from build123d import *

# Parameters (mm, degrees)
F0_R      = 2.0455133379
F0_R_2    = 1.5
F1_DEPTH  = 20
F0_W      = 30
F0_H      = 6.4
F2_DEPTH  = 30
F3_R      = 6.5
F4_DEPTH  = 18.001
F5_R      = 3
F5_R_2    = 2.0455133379
F6_DEPTH  = 15
F7_R      = 9.25
F8_DEPTH  = 20.001
F9_DEPTH  = 10
F11_DEPTH = 3


with BuildPart() as f1:
    # F0 (on Top) → F1 (new body)
    with BuildSketch(Plane.XY):
        Polygon((11.3, 6.4), (0, 6.4), (-27.3, 6.4), (-27.3, -6.4), (-11, -6.4), (-11, -4.4), (0, -4.4), (11, -4.4), (11, -6.4), (27.3, -6.4), (27.3, 0), (27.3, 13.6), (11.3, 13.6), align=None)
        with Locations((-21, -0.9)):
            Circle(F0_R, mode=Mode.SUBTRACT)
        with Locations((-9, 1.4)):
            Circle(F0_R_2, mode=Mode.SUBTRACT)
        with Locations((9, 1.4)):
            Circle(F0_R_2, mode=Mode.SUBTRACT)
        with Locations((21, -0.9)):
            Circle(F0_R, mode=Mode.SUBTRACT)
    extrude(amount=F1_DEPTH)

    # F0 (on Top) → F2 (join)
    with BuildSketch(Plane.XY):
        with Locations((42.3, -3.2)):
            Rectangle(F0_W, F0_H)
    extrude(amount=F2_DEPTH)

    # F3 (on face) → F4 (cut, through all)
    with BuildSketch(Plane.XZ.offset(4.4)):
        with Locations((0, 20)):
            Circle(F3_R)
    extrude(amount=-F4_DEPTH, mode=Mode.SUBTRACT)

    # F5 (on face) → F6 (cut)
    with BuildSketch(Plane(origin=(0, 0, 0), x_dir=(1, 0, 0), z_dir=(0, 0, -1))):
        with Locations((-21, 0.9)):
            Circle(F5_R)
        with Locations((-21, 0.9)):
            Circle(F5_R_2, mode=Mode.SUBTRACT)
        with Locations((21, 0.9)):
            Circle(F5_R)
        with Locations((21, 0.9)):
            Circle(F5_R_2, mode=Mode.SUBTRACT)
    extrude(amount=-F6_DEPTH, mode=Mode.SUBTRACT)

    # F7 (on face) → F8 (cut, through all)
    with BuildSketch(Plane.XZ.offset(6.4)):
        with Locations((42.3, 15)):
            Circle(F7_R)
    extrude(amount=-F8_DEPTH, mode=Mode.SUBTRACT)

    # F9 (cut): a face of the model
    f9_faces = [f1.faces().sort_by_distance(p)[0] for p in [
        (42.3, -3.2, 30),
    ]]
    extrude(f9_faces, amount=-F9_DEPTH, mode=Mode.SUBTRACT)

    # F10 (on face) → F11 (cut)
    with BuildSketch(Plane.XY):
        Polygon((12, 1.4), (10.5, 3.9980762114), (7.5, 3.9980762114), (6, 1.4), (7.5, -1.1980762114), (10.5, -1.1980762114), align=None)
        Polygon((-10.5, -1.1980762114), (-7.5, -1.1980762114), (-6, 1.4), (-7.5, 3.9980762114), (-10.5, 3.9980762114), (-12, 1.4), align=None)
    extrude(amount=F11_DEPTH, mode=Mode.SUBTRACT)


solid = f1.part
Verification items for the finished model (mm, model axes). A direction names the side the tool comes from. Coordinates: 2 decimals unless noted, no trailing zeros. Loops run counter-clockwise (first coordinate to the right, second up) from the corner with the lowest first, then second, coordinate; pieces in that order, holes last. Notation, with made-up numbers: M 34,66.5 L 74,66.5 A8 cw 74,71.5 Z; hole C -32,71 d5. An arc over 180 degrees is marked long. One line per item, written item: value.
1. Section check C-C on z = 2. Record the cut outline in (x, y), plus the area to 3 significant figures.
Answers follow:
outline: M -27.3,-6.4 L -11,-6.4 L -11,-4.4 L 11,-4.4 L 11,-6.4 L 57.3,-6.4 L 57.3,0 L 27.3,0 L 27.3,13.6 L 11.3,13.6 L 11.3,6.4 L -27.3,6.4 Z; hole C -21,-0.9 d6; hole M -12,1.4 L -10.5,-1.2 L -7.5,-1.2 L -6,1.4 L -7.5,4 L -10.5,4 Z; hole M 6,1.4 L 7.5,-1.2 L 10.5,-1.2 L 12,1.4 L 10.5,4 L 7.5,4 Z; hole C 21,-0.9 d6
area: 859 mm^2
2. Set-up check for faces 4 (the flat face through (27.3, 7, 10)), 5 (the flat face through (-11, -5, 10)), 6 (the flat face through (-19, -2, 15)), 7 (the flat face through (29, -6.4, 8)): record each of +Z, -Z, +X, -X, +Y, -Y from which the full face is reachable in a straight line by a thin tool's end or side.
Answers follow:
face 4: +Z, -Z, +X, +Y
face 5: +Z, -Z, -Y
face 6: -Z
face 7: +Z, -Z, +X, -X, -Y
3. Mould release check, pull along X, two halves, no side actions. Record for faces 1 (the flat face through (54, -3, 20)), 2 (the flat face through (-8, 3, 3)), 3 (the flat face through (57.3, -3, 10)): pulls with the +X half, pulls with the -X half, needs draft (parallel to the pull), parting line crosses it, or undercut.
Answers follow:
face 1: needs draft
face 2: undercut
face 3: pulls with the +X half
4. Section check B-B on x = 21. Record the cut outline in (y, z).
Answers follow:
outline: M -6.4,0 L -3.9,0 L -3.9,15 L -2.95,15 L -2.95,20 L -6.4,20 Z; M 1.15,15 L 2.1,15 L 2.1,0 L 13.6,0 L 13.6,20 L 1.15,20 Z
5. Material ranges on line 1 along Y through (x, z) = (21, 18); line 2 along Y through (x, z) = (9, 14); line 3 along X through (y, z) = (-0.9, 11.25), recorded low to high. Write a range as from..to.
Answers follow:
line 1: -6.4..-2.95, 1.15..13.6
line 2: -4.4..-0.1, 2.9..6.4
line 3: -27.3..-24, -18..18, 24..33.84, 50.76..57.3
6. Section check D-D on x = 9. Record the cut outline in (y, z), plus the area to 3 significant figures.
Answers follow:
outline: M -4.4,0 L -1.2,0 L -1.2,3 L -0.1,3 L -0.1,20 L -4.4,20 Z; M 2.9,3 L 4,3 L 4,0 L 6.4,0 L 6.4,20 L 2.9,20 Z
area: 149 mm^2
7. Section check A-A on z = 10. Record the cut outline in (x, y), plus the area to 3 significant figures.
Answers follow:
outline: M -27.3,-6.4 L -11,-6.4 L -11,-4.4 L 11,-4.4 L 11,-6.4 L 34.52,-6.4 L 34.52,0 L 27.3,0 L 27.3,13.6 L 11.3,13.6 L 11.3,6.4 L -27.3,6.4 Z; M 50.08,-6.4 L 57.3,-6.4 L 57.3,0 L 50.08,0 Z; hole C -21,-0.9 d6; hole C -9,1.4 d3; hole C 9,1.4 d3; hole C 21,-0.9 d6
area: 792 mm^2
8. Gauge pin test, flat ends, axial feed: P1, Ø1.5, axis at y = 2, z = 16, coming from the +X side; P2, Ø4, axis at x = 20, y = -1.5, coming from the +Z side; P3, Ø1, axis at x = 9, z = 8, coming from the -Y side; P4, Ø2.5, axis at x = -9.5, z = 1, coming from the +Y side. Record the tip position at first contact, or that the pin passes through.
Answers follow:
P1: x = 27.3
P2: z = 20
P3: y = -4.4
P4: y = 6.4
